from build123d import *

# Parameters (mm, degrees)
F0_R     = 12
F0_R_2   = 11
F0_R_3   = 5
F0_R_4   = 4.1
F0_R_5   = 3
F1_DEPTH = 2
F2_DEPTH = 3.5
F3_SIZE  = 0.99999
F4_DEPTH = 4.5
F5_DEPTH = 7.5
F6_DEPTH = 10
F7_SIZE  = 1
F8_SIZE  = 0.5


# Not quite as in the source:
# - a fillet or chamfer is up to 0.001 mm smaller than in the source, because OpenCascade refuses the exact size


with BuildPart() as f1:
    # F0 (on Top) → F1 (new body)
    with BuildSketch(Plane.XY):
        Circle(F0_R)
        Circle(F0_R_2, mode=Mode.SUBTRACT)
        Circle(F0_R_2)
        Circle(F0_R_3, mode=Mode.SUBTRACT)
        Circle(F0_R_3)
        Circle(F0_R_4, mode=Mode.SUBTRACT)
        Circle(F0_R_4)
        Circle(F0_R_5, mode=Mode.SUBTRACT)
        Circle(F0_R_5)
    extrude(amount=F1_DEPTH)

    # F0 (on Top) → F2 (join)
    with BuildSketch(Plane.XY):
        Circle(F0_R_2)
        Circle(F0_R_3, mode=Mode.SUBTRACT)
        Circle(F0_R_3)
        Circle(F0_R_4, mode=Mode.SUBTRACT)
        Circle(F0_R_4)
        Circle(F0_R_5, mode=Mode.SUBTRACT)
        Circle(F0_R_5)
    extrude(amount=F2_DEPTH)

    # F3 (size 1 in the source; OpenCascade refuses exactly that, so slightly less here)
    f3_edges = [f1.edges().sort_by_distance(p)[0] for p in [
        (-11, 0, 2),
    ]]
    chamfer(f3_edges, length=F3_SIZE)

    # F0 (on Top) → F4 (join)
    with BuildSketch(Plane.XY):
        Circle(F0_R_3)
        Circle(F0_R_4, mode=Mode.SUBTRACT)
        Circle(F0_R_4)
        Circle(F0_R_5, mode=Mode.SUBTRACT)
        Circle(F0_R_5)
    extrude(amount=F4_DEPTH)

    # F0 (on Top) → F5 (join)
    with BuildSketch(Plane.XY):
        Circle(F0_R_4)
        Circle(F0_R_5, mode=Mode.SUBTRACT)
    extrude(amount=F5_DEPTH)

    # F0 (on Top) → F6 (join)
    with BuildSketch(Plane.XY):
        Circle(F0_R_5)
    extrude(amount=F6_DEPTH)

    # F7
    f7_edges = [f1.edges().sort_by_distance(p)[0] for p in [
        (-12, 0, 0),
    ]]
    chamfer(f7_edges, length=F7_SIZE)

    # F8
    f8_edges = [f1.edges().sort_by_distance(p)[0] for p in [
        (-11, 0, 3.5),
    ]]
    chamfer(f8_edges, length=F8_SIZE)


solid = f1.part
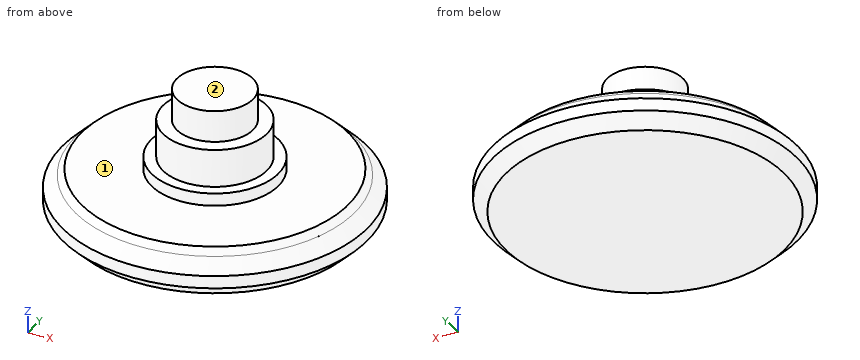
Read the model definition and answer for the solid it produces. Units are mm, in the model's axes. Face numbers are marked on the shaded views. A direction names the side the tool comes from. Round coordinates to 2 decimals unless told otherwise and drop trailing zeros. Write each loop counter-clockwise with the first axis right and the second up, starting at its lowest first coordinate (ties: lowest second). Pieces come first, ordered by that corner, then holes. Notation, with made-up numbers: M 69.25,73.25 L 97.25,73.25 A6 ccw 97.25,82.25 Z; hole C 57,-25.5 d5. An arc over 180 degrees is marked long. Use a Markdown table: item, result.
1) Straight lines are drawn through the part: line 1 along Z through (x, y) = (9.5, 4); line 2 along Z through (x, y) = (-2.5, 4); line 3 along Y through (x, z) = (-3.5, 6). For each, find the intervals that lie inside material, in ascending order. Write a range as [from, to].
Answers follow:
| item | result |
|---|---|
| line 1 | z = [0, 3.5] |
| line 2 | z = [0, 4.5] |
| line 3 | y = [-2.14, 2.14] |
2) A tool of negligible diameter and unlimited length cuts with its end or side. For the marked faces 1 and 2, from which of +Z, -Z, +X, -X, +Y, -Y can it reach the whole face along a straight path? Write none if from no direction.
Answers follow:
| item | result |
|---|---|
| face 1 | +Z |
| face 2 | +Z, +X, -X, +Y, -Y |
3) The part is cut by section C-C (z = 5). Write down the section's boundary in (x, y).
Answers follow:
| item | result |
|---|---|
| outline | C 0,0 d8.2 |
4) The part is cut by section D-D (z = 8). Write down the section's boundary in (x, y), plus the area to 3 significant figures.
Answers follow:
| item | result |
|---|---|
| outline | C 0,0 d6 |
| area | 28.3 mm2 |
5) Flat-ended cylindrical pins translate along their axes: pin 1 (1.5 mm diameter, centred on y = -0.5, z = 6, fed in from +X); pin 2 (4 mm diameter, centred on x = 5.5, y = -6, fed in from +Z); pin 3 (6 mm diameter, centred on x = -6, z = 1, fed in from +Y); pin 4 (6 mm diameter, centred on x = 2, y = -5.5, fed in from -Z). Find the tip coordinate at first contact, or state that the pin passes through.
Answers follow:
| item | result |
|---|---|
| pin 1 | stops at x = 4.1 |
| pin 2 | stops at z = 3.5 |
| pin 3 | stops at y = 11.62 |
| pin 4 | stops at z = 0 |
